Source: CAD feature listing. Evaluate the final solid. Frame: model axes, mm. A direction names the side the tool comes from. Give positions to 0.01 mm unless a question says otherwise; leave off trailing zeros. Order: outer loops, then holes, each group sorted by start corner. A loop starts at its lowest first (then second) coordinate and runs counter-clockwise, first axis right, second up. Notation, with made-up numbers: M 18,-11 L 28,-11 A8 ccw 28,-7 Z; hole C 77.25,80.5 d1. An arc over 180 degrees is marked long. Answer as a JSON object with one key per item and string values. Group by question number.
1. Material intervals for L1, parallel to Z at x = -6.5, y = 1.85; L2, parallel to Z at x = -12.5, y = 1.85; L3, parallel to Z at x = -11, y = 1.8, sorted ascending. Write a range as [from, to].
2. Pin query (flat end, axial travel): P1, Ø0.5, axis at y = 2.5, z = 40, coming from the -X side; P2, Ø3, axis at x = -7.5, z = 39.5, coming from the +Y side; P3, Ø0.8, axis at x = -12, y = 2.5, coming from the +Z side; P4, Ø0.5, axis at y = 2.5, z = 39.5, coming from the +X side. Return the tip coordinate at first contact, or that it passes through.
3. Section query A-A (z = 41). Output: boundary loops of the cut face in (x, y).
4. Section query C-C (y = 1.65). Output: boundary loops of the cut face in (x, z), plus the area to 3 significant figures.
5. Set-up query: faces 4 (the flat face through (-10.8, 2.5, 41.582)), 5 (the flat face through (-13.594, 2.5, 40.1)), 6 (the flat face through (-8.096, 2.5, 40.1)), 7 (the flat face through (-10.9, 2.5, 38.663)), 8 (the flat face through (-11, 3, 40)). Return all of +Z, -Z, +X, -X, +Y, -Y with unobstructed straight access to the full face (end or side cutting, diameter ignored); none if empty.
6. Section query D-D (x = -9). Output: boundary loops of the cut face in (y, z), plus the area to 3 significant figures.
7. Section query B-B (x = -7.75). Output: boundary loops of the cut face in (y, z), plus the area to 3 significant figures.
8. Pull-direction query (X, two-part tool) for faces 1 (the flat face through (-4.308, 1, 38)), 2 (the flat face through (-14.708, 1, 38)), 3 (the cylindrical face through (-6.584, 1.189, 32.468)); classes: +X half, -X half, draft (parallel to the pull), parting line (faces both ways), or undercut.
Autodesk Inventor part; units mm, degrees
ref_plane "YZ Plane" through (0, 0, 0) normal (1, 0, 0) x (0, 1, 0)
ref_plane "XZ Plane" through (0, 0, 0) normal (0, 1, 0) x (-1, 0, 0)
ref_plane "XY Plane" through (0, 0, 0) normal (0, 0, 1) x (1, 0, 0)
sketch "Sketch1" plane through (0, 0, 0) normal (0, 1, 0) x (-1, 0, 0)
  line L0 (14.7075, 31.6187) -> (4.3075, 31.6187)
  line L1 (4.3075, 31.6187) -> (4.3075, 44.7187)
  line L2 (4.3075, 44.7187) -> (14.7075, 44.7187)
  line L3 (14.7075, 44.7187) -> (14.7075, 31.6187)
  line L4 (13.5937, 38.6629) -> (8.0964, 38.6629)
  line L5 (8.0964, 38.6629) -> (8.0964, 41.5823)
  line L6 (8.0964, 41.5823) -> (13.5937, 41.5823)
  line L7 (13.5937, 41.5823) -> (13.5937, 38.6629)
  circle A0 centre (6.5746, 42.8557) radius 1.4817
  point P0 (0, 0)
  dimension "d0" = 10.4
  dimension "d1" = 13.1
extrude "Extrusion1" add sketch "Sketch1" along normal blind 2
extrude "Extrusion2" add sketch "Sketch1" along normal blind 3 contours L4 L5 L6 L7
sketch "Sketch2" plane through (0, 2, 0) normal (0, 1, 0) x (1, 0, 0)
  line L0 (-13.674, -32.9177) -> (-5.5891, -32.9177)
  line L1 (-13.5937, -43.2778) -> (-9.2456, -43.2778)
  point P0 (0, 0)
  point P1 (-13.0646, -32.9177)
  point P2 (-6.5641, -32.9177)
  point P3 (-10.952, -32.9177)
  point P4 (-8.8393, -32.9177)
  point P5 (-12.5364, -43.2778)
  point P6 (-10.3019, -43.2778)
hole "Hole1" at (-13.0646, 2, 32.9177) at (-6.5641, 2, 32.9177) at (-10.952, 2, 32.9177) at (-8.8393, 2, 32.9177) at (-12.5364, 2, 43.2778) at (-10.3019, 2, 43.2778) direction (0, -1, 0) diameter 0.9 end through all
sketch "Sketch3" plane through (0, 0, 0) normal (0, -1, 0) x (1, 0, 0)
  circle A0 centre (-12.5364, 43.2778) radius 0.45
  circle A1 centre (-10.952, 32.9177) radius 0.45
  circle A2 centre (-13.0646, 32.9177) radius 0.45
  circle A3 centre (-6.5641, 32.9177) radius 0.45
  circle A4 centre (-8.8393, 32.9177) radius 0.45
  circle A5 centre (-10.3019, 43.2778) radius 0.45
  line L0 (-14.7075, 44.7187) -> (-4.3075, 44.7187)
  line L1 (-14.7075, 31.6187) -> (-14.7075, 44.7187)
  line L2 (-4.3075, 31.6187) -> (-14.7075, 31.6187)
  line L3 (-4.3075, 44.7187) -> (-4.3075, 31.6187)
  circle A6 centre (-6.5746, 42.8557) radius 1.4817
  point P0 (0, 0)
extrude "Extrusion3" cut sketch "Sketch3" against normal blind 0.4
sketch "Sketch4" plane through (-13.5937, 2, 41.5823) normal (0, 0, 1) x (1, 0, 0)
  line L0 (5.4973, 0) -> (0, 0)
  line L1 (5.4973, 0) -> (5.4973, 1)
  line L2 (0, 1) -> (5.4973, 1)
  line L3 (0, 0) -> (0, 1)
  line L4 (9.2862, 0) -> (-1.1138, 0)
  line L5 (2.7486, 0) -> (2.7486, 3.0289)
  line L6 (2.7486, 0) -> (3.8152, 4.8108)
  line L7 (2.7486, 0) -> (1.9494, 3.6052)
  line L8 (3.8152, 4.8108) -> (52.0967, 222.5946)
  line L9 (1.9494, 3.6052) -> (-46.5994, 222.5946)
  arc A0 (52.0967, 222.5946) -> (-46.5994, 222.5946) centre (2.7486, 0) ccw
  point P0 (13.5937, -2)
  dimension "d15" = 12.5
  dimension "d16" = 12.5
properties part number "tof"
Answer sheet:
{
 "1": {"L1": "[31.62, 32.47], [33.36, 41.38], [44.34, 44.72]", "L2": "[31.62, 42.83], [43.73, 44.72]", "L3": "[31.62, 32.47], [33.37, 44.72]"},
 "2": {"P1": "x = -13.59", "P2": "y = 3", "P3": "z = 41.58", "P4": "x = -8.1"},
 "3": {"outline": "M -14.71,0.4 L -4.31,0.4 L -4.31,2 L -8.1,2 L -8.1,3 L -13.59,3 L -13.59,2 L -14.71,2 Z"},
 "4": {"outline": "M -14.71,31.62 L -4.31,31.62 L -4.31,44.72 L -14.71,44.72 Z; hole C -13.06,32.92 d0.9; hole C -12.54,43.28 d0.9; hole C -10.95,32.92 d0.9; hole C -10.3,43.28 d0.9; hole C -8.84,32.92 d0.9; hole C -6.57,42.86 d2.96; hole C -6.56,32.92 d0.9", "area": "126 mm^2"},
 "5": {"face 4": "+Z, +X, -X, +Y", "face 5": "+Z, -Z, -X, +Y", "face 6": "+Z, -Z, +X, +Y", "face 7": "-Z, +X, -X, +Y", "face 8": "+Z, -Z, +X, -X, +Y"},
 "6": {"outline": "M 0.4,31.62 L 2,31.62 L 2,32.5 L 0.4,32.5 Z; M 0.4,33.34 L 2,33.34 L 2,38.66 L 3,38.66 L 3,41.58 L 2,41.58 L 2,44.72 L 0.4,44.72 Z", "area": "22.5 mm^2"},
 "7": {"outline": "M 0.4,31.62 L 2,31.62 L 2,41.95 L 0.4,41.95 Z; M 0.4,43.76 L 2,43.76 L 2,44.72 L 0.4,44.72 Z", "area": "18.1 mm^2"},
 "8": {"face 1": "+X half", "face 2": "-X half", "face 3": "undercut"}
}
